from build123d import *

# Parameters (mm, degrees)
F1_DEPTH = 3
F2_COUNT = 4
F2_ANGLE = 270
F3_R     = 5
F4_DEPTH = 3


with BuildPart() as f1:
    # F0 (on Top) → F1 (new body)
    with BuildSketch(Plane.XY):
        with BuildLine():
            Line((0, 25), (0, 0))
            Line((0, 0), (24.620194, 4.341204))
            ThreePointArc((24.620194, 4.341204), (23.629844, 15.660952), (12.310097, 14.670602))
            ThreePointArc((12.310097, 14.670602), (11.319747, 25.99035), (0, 25))
        make_face()
    extrude(amount=F1_DEPTH)



with BuildPart() as f2_1:
    # F2: instance of F1
    add(f1.part.rotate(Axis((0, 0, 1.5), (0, 0, 1)), 1 * F2_ANGLE / (F2_COUNT - 1)))


with BuildPart() as f2_2:
    # F2: instance of F1
    add(f1.part.rotate(Axis((0, 0, 1.5), (0, 0, 1)), 2 * F2_ANGLE / (F2_COUNT - 1)))


with BuildPart() as f2_3:
    # F2: instance of F1
    add(f1.part.rotate(Axis((0, 0, 1.5), (0, 0, 1)), 3 * F2_ANGLE / (F2_COUNT - 1)))


with BuildPart() as f1_1:
    add(f1.part)

    add(f2_1.part)  # F4 merges F2_1

    add(f2_2.part)  # F4 merges F2_2

    add(f2_3.part)  # F4 merges F2_3
    # F3 (on Top) → F4 (join)
    with BuildSketch(Plane.XY):
        Circle(F3_R)
    extrude(amount=F4_DEPTH)


solid = f1_1.part
Verification items for the finished model (mm, model axes). A direction names the side the tool comes from. Coordinates: 2 decimals unless noted, no trailing zeros. Loops run counter-clockwise (first coordinate to the right, second up) from the corner with the lowest first, then second, coordinate; pieces in that order, holes last. Notation, with made-up numbers: (-15, 67) -> (-5, 67) arc R28 ccw to (-5, 88) -> close; hole circle Ø1 at (37, -4.75). An arc over 180 degrees is marked (long way). Answer as a JSON object with one key per item and string values. Group by question number.
Item 1: Scan lines: probe 1 along X at (y, z) = (15.5, 1.1); probe 2 along Y at (x, z) = (19, 2.45); probe 3 along X at (y, z) = (-13, 2.75). Record each from-to range of solid material in increasing order.
Item 2: Tool access check on faces 4 (the flat face through (-15, 0, 1)), 5 (the flat face through (15, 0, 1)), 6 (the flat face through (0, 15, 1)), 7 (the flat face through (0, -15, 1)). Record the directions out of +Z, -Z, +X, -X, +Y, -Y that give a thin tool (end or side, any length) a straight path to the whole face; none if there is none.
Item 3: Sectioned sample at B-B on x = -16. Record the boundary of the cut face in (y, z), plus the area to 3 significant figures.
Item 4: Sectioned sample at D-D on x = 9.5. Record the boundary of the cut face in (y, z).
Item 5: Sectioned sample at A-A on y = -10.5. Record the boundary of the cut face in (x, z), plus the area to 3 significant figures.
Item 6: Depth check by flat-ended pin: pin 1 (1 mm diameter, centred on x = -20.5, y = -9, fed in from -Z); pin 2 (1.5 mm diameter, centred on x = -11, z = 1.5, fed in from -Y). Enter the tip coordinate at first touch or a pass-through.
Item 7: Sectioned sample at C-C on z = 0.45. Record the boundary of the cut face in (x, y), plus the area to 3 significant figures.
Item 8: Mould release check, pull along X, two halves, no side actions. Record for faces 1 (the cylindrical face through (25.88, -11.45, 1.48)), 2 (the flat face through (14.63, 2.58, 1.48)), 3 (the flat face through (0, 0, 0)): +X half, -X half, draft (parallel to the pull), parting line (faces both ways), or undercut.
Evaluation:
{
 "1": {"probe 1": "x = -16.97 to -2.73, 0 to 12.92, 13.11 to 23.82", "probe 2": "y = -14.15 to 0, 3.35 to 17.52", "probe 3": "x = -25.7 to 0, 2.29 to 15.4, 15.63 to 24.04"},
 "2": {"face 4": "+Z, -Z, -X", "face 5": "+Z, -Z, +X", "face 6": "+Z, -Z, +Y", "face 7": "+Z, -Z, -Y"},
 "3": {"outline": "(-17.15, 0) -> (-2.82, 0) -> (-2.82, 3) -> (-17.15, 3) -> close; (0, 0) -> (13.22, 0) -> (13.22, 3) -> (0, 3) -> close; (13.73, 0) -> (23.2, 0) -> (23.2, 3) -> (13.73, 3) -> close", "area": "111 mm²"},
 "4": {"outline": "(-26.5, 0) -> (0, 0) -> (0, 3) -> (-26.5, 3) -> close; (1.68, 0) -> (27.14, 0) -> (27.14, 3) -> (1.68, 3) -> close"},
 "5": {"outline": "(-26.44, 0) -> (0, 0) -> (0, 3) -> (-26.44, 3) -> close; (1.85, 0) -> (26.59, 0) -> (26.59, 3) -> (1.85, 3) -> close", "area": "154 mm²"},
 "6": {"pin 1": "stops at z = 0", "pin 2": "stops at y = -26.75"},
 "7": {"outline": "(-25, 0) -> (-5, 0) arc R5 ccw to (-4.92, -0.87) -> (-24.62, -4.34) arc R8.03 ccw to (-12.31, -14.67) arc R8.03 ccw to (0, -25) -> (0, -5) arc R5 ccw to (0.87, -4.92) -> (4.34, -24.62) arc R8.03 ccw to (14.67, -12.31) arc R8.03 ccw to (25, 0) -> (5, 0) arc R5 ccw to (4.92, 0.87) -> (24.62, 4.34) arc R8.03 ccw to (12.31, 14.67) arc R8.03 ccw to (0, 25) -> (0, 5) arc R5 ccw to (-0.87, 4.92) -> (-4.34, 24.62) arc R8.03 ccw to (-14.67, 12.31) arc R8.03 ccw to start", "area": "2,050 mm²"},
 "8": {"face 1": "undercut", "face 2": "+X half", "face 3": "draft"}
}
